Could you check a few things on this drawing? It's one solid part, dimensions in mm from its lowest x, y, z. A direction names the side the tool comes from. Give positions to 0.01 mm unless a question says otherwise; leave off trailing zeros. Order: outer loops, then holes, each group sorted by start corner. A loop starts at its lowest first (then second) coordinate and runs counter-clockwise, first axis right, second up.
Item 1: I want a section at D-D, the plane y = 6.5. Write out the boundary of the cut face in (x, z), then the cut area to 3 significant figures.
Item 2: I want a section at A-A, the plane y = 45. Write out the boundary of the cut face in (x, z), then the cut area to 3 significant figures.
Item 3: If I drill on line 1 along X through (y, z) = (37, 12); line 2 along Y through (x, z) = (56, 6.5); line 3 along Z through (x, y) = (6, 7.5), over which ranges is the centre line in solid material (lowest first)?
Item 4: I want a section at B-B, the plane z = 6.25. Write out the boundary of the cut face in (x, y).
Item 5: Which directions (+Z, -Z, +X, -X, +Y, -Y) give clear straight access to the entire face, cutting with the end or side of a thin tool? Please do the marked faces 1, 2 and 3.
Item 6: I'm going to push flat-ended pins straight in: pin 1 Ø8 at (x, y) = (3, 24) entering from +Z; pin 2 Ø0.9 at (y, z) = (23.5, 23.5) entering from +X; pin 3 Ø0.9 at (y, z) = (20.5, 24) entering from -X. Where does each tip first touch, or does it pass through?
Item 7: I want a section at C-C, the plane x = 65. Write out the boundary of the cut face in (y, z), then the cut area to 3 significant figures.
Item 8: If we mould it in two halves opening along Y, with no side actions, what happens to the marked faces 4, 5 and 6? For each: +Y half, -Y half, draft (parallel to the pull), parting line (faces both ways), or undercut.
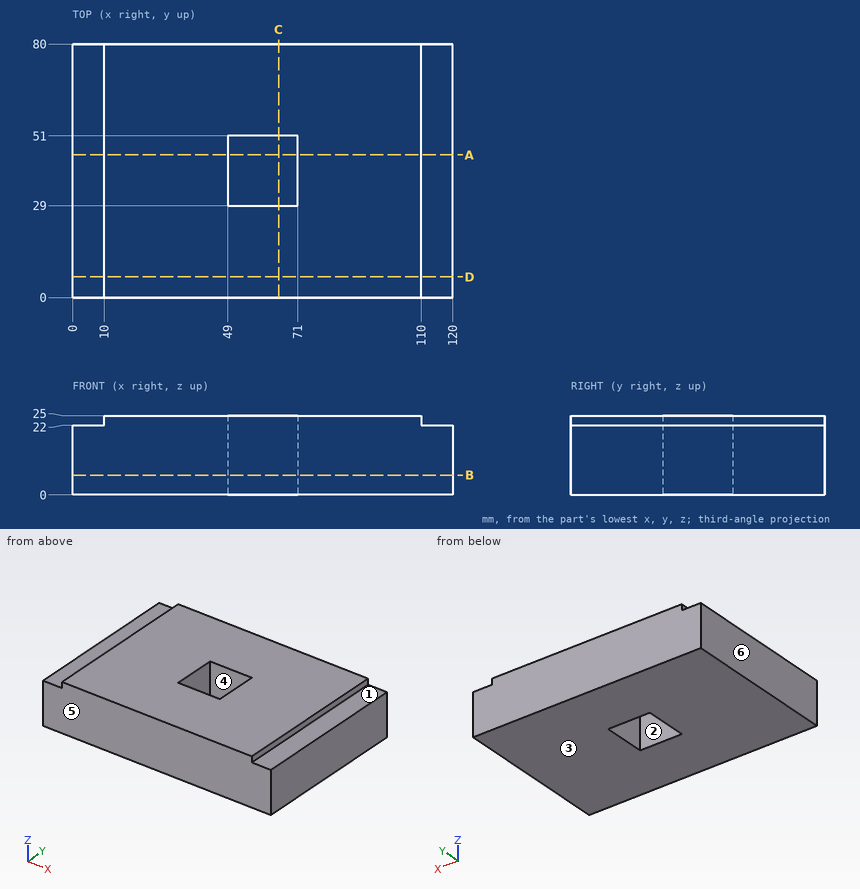
Results list:
1. outline: (0, 0) - (120, 0) - (120, 22) - (110, 22) - (110, 25) - (10, 25) - (10, 22) - (0, 22) - close
1. area: 2,940 mm2
2. outline: (0, 0) - (49, 0) - (49, 25) - (10, 25) - (10, 22) - (0, 22) - close; (71, 0) - (120, 0) - (120, 22) - (110, 22) - (110, 25) - (71, 25) - close
2. area: 2,390 mm2
3. line 1: x = 0 to 49, 71 to 120
3. line 2: y = 0 to 29, 51 to 80
3. line 3: z = 0 to 22
4. outline: (0, 0) - (120, 0) - (120, 80) - (0, 80) - close; hole (49, 29) - (71, 29) - (71, 51) - (49, 51) - close
5. face 1: +Z, +X, +Y, -Y
5. face 2: +Z, -Z
5. face 3: -Z, +X, -X, +Y, -Y
6. pin 1: stops at z = 22
6. pin 2: stops at x = 110
6. pin 3: stops at x = 10
7. outline: (0, 0) - (29, 0) - (29, 25) - (0, 25) - close; (51, 0) - (80, 0) - (80, 25) - (51, 25) - close
7. area: 1,450 mm2
8. face 4: undercut
8. face 5: -Y half
8. face 6: draft
